```python
from build123d import *

# Parameters (mm, degrees)
SKIZZE1_R                       = 400
AUFSATZ_LINEAR_AUSTRAGEN1_DEPTH = 300
SCHNITT_LINEAR_AUSTRAGEN1_DEPTH = 25
SCHNITT_LINEAR_AUSTRAGEN2_DEPTH = 25
SCHNITT_LINEAR_AUSTRAGEN3_DEPTH = 25


with BuildPart() as part:
    # Skizze1 → Aufsatz-Linear austragen1 (new body, symmetric)
    with BuildSketch(Plane.XY):
        Circle(SKIZZE1_R)
    extrude(amount=AUFSATZ_LINEAR_AUSTRAGEN1_DEPTH, both=True)

    # Skizze2 → Schnitt-Linear austragen1 (cut, symmetric)
    with BuildSketch(Plane.XY.offset(200)):
        with BuildLine():
            Line((0, 400), (0, 340))
            Line((0, 340), (-210.713075057, 340))
            ThreePointArc((-210.713075057, 340), (-109.544511501, 384.707681233), (0, 400))
        make_face()
    extrude(amount=SCHNITT_LINEAR_AUSTRAGEN1_DEPTH, both=True, mode=Mode.SUBTRACT)

    # Skizze3 → Schnitt-Linear austragen2 (cut, symmetric)
    with BuildSketch(Plane.XY.offset(100)):
        with BuildLine():
            Line((-136.80805733, 375.877048314), (-116.286848731, 319.495491067))
            Line((-116.286848731, 319.495491067), (-314.292370465, 247.427374936))
            ThreePointArc((-314.292370465, 247.427374936), (-234.515945379, 324.040539691), (-136.80805733, 375.877048314))
        make_face()
    extrude(amount=SCHNITT_LINEAR_AUSTRAGEN2_DEPTH, both=True, mode=Mode.SUBTRACT)

    # Skizze4 → Schnitt-Linear austragen3 (cut, symmetric)
    with BuildSketch(Plane.XY):
        with BuildLine():
            Line((-257.115043875, 306.417777248), (-218.547787293, 260.45511066))
            Line((-218.547787293, 260.45511066), (-379.963367533, 125.011356815))
            ThreePointArc((-379.963367533, 125.011356815), (-331.201295158, 224.289326732), (-257.115043875, 306.417777248))
        make_face()
    extrude(amount=SCHNITT_LINEAR_AUSTRAGEN3_DEPTH, both=True, mode=Mode.SUBTRACT)


solid = part.part
```
Input: part model. Units: mm. Frame: model coordinates. A direction names the side the tool comes from. Coordinates: 2 decimals unless noted, no trailing zeros. Loops run counter-clockwise (first coordinate to the right, second up) from the corner with the lowest first, then second, coordinate; pieces in that order, holes last. Notation, with made-up numbers: (28.25, -33.5) - (38.25, -33.5) arc R26 cw to (38.25, -7.5) - close; hole circle Ø4 at (-32.75, 27). An arc over 180 degrees is marked (long way). Answer in a Markdown table with one row per item.
(1) Mould query, pull axis Y, two halves, no side actions, for faces 4 (the face through (-293, 223, -25)), 5 (the face through (-104, 340, 200)), 6 (the face through (-80, 364, 175)). Classes: pulls with the +Y half, pulls with the -Y half, needs draft (parallel to the pull), parting line crosses it, or undercut.
Model answer:
| item | result |
|---|---|
| face 4 | undercut |
| face 5 | pulls with the +Y half |
| face 6 | needs draft |
(2) Cut plane C-C on y = -181. Output: boundary loops of the cut face in (x, z), plus the area to 3 significant figures.
Model answer:
| item | result |
|---|---|
| outline | (-356.71, -300) - (356.71, -300) - (356.71, 300) - (-356.71, 300) - close |
| area | 428,000 mm² |
(3) Cut plane B-B on x = 307. Output: boundary loops of the cut face in (y, z).
Model answer:
| item | result |
|---|---|
| outline | (-256.42, -300) - (256.42, -300) - (256.42, 300) - (-256.42, 300) - close |
(4) Cut plane D-D on z = -160. Output: boundary loops of the cut face in (x, y), plus the area to 3 significant figures.
Model answer:
| item | result |
|---|---|
| outline | circle Ø800 at (0, 0) |
| area | 503,000 mm² |
(5) Pin query (flat end, axial travel): P1, Ø1, axis at y = 312.5, z = 202, coming from the -X side; P2, Ø6, axis at y = -245.5, z = -207.5, coming from the -X side; P3, Ø12, axis at y = -276.5, z = 8, coming from the +X side. Return the tip coordinate at first contact, or that it passes through.
Model answer:
| item | result |
|---|---|
| P1 | stops at x = -250.31 |
| P2 | stops at x = -318.11 |
| P3 | stops at x = 294.67 |
(6) Material intervals for L1, parallel to Z at x = -160, y = 346; L2, parallel to Y at x = -320.5, z = 152.5; L3, parallel to X at y = 160, z = 105.5, sorted ascending. Write a range as from..to.
Model answer:
| item | result |
|---|---|
| L1 | z = -300..75, 125..175, 225..300 |
| L2 | y = -239.33..239.33 |
| L3 | x = -366.61..366.61 |
(7) Set-up query: faces 1 (the face through (-80, 364, 225)), 2 (the face through (-6, 6, 300)), 3 (the face through (-126.7, 348.1, 100.4)). Return all of +Z, -Z, +X, -X, +Y, -Y with unobstructed straight access to the full face (end or side cutting, diameter ignored); none if empty.
Model answer:
| item | result |
|---|---|
| face 1 | -X, +Y |
| face 2 | +Z, +X, -X, +Y, -Y |
| face 3 | -X |
(8) Cut plane A-A on z = -8. Output: boundary loops of the cut face in (x, y), plus the area to 3 significant figures.
Model answer:
| item | result |
|---|---|
| outline | (-379.96, 125.01) arc R400 ccw (long way) to (-257.12, 306.42) - (-218.55, 260.46) - close |
| area | 494,000 mm² |
